Read the model definition and answer for the solid it produces. Units are mm, in the model's axes. A direction names the side the tool comes from. Give positions to 0.01 mm unless a question says otherwise; leave off trailing zeros. Loops run counter-clockwise (first coordinate to the right, second up) from the corner with the lowest first, then second, coordinate; pieces in that order, holes last.
(1) Find section C-C, the plane x = 1.5. Write down the section's boundary in (y, z), then the cut area to 3 significant figures.
(2) Find section A-A, the plane x = 6.75. Write down the section's boundary in (y, z), then the cut area to 3 significant figures.
(3) Straight lines are drawn through the part: probe 1 along Y at (x, z) = (15.95, 11.5); probe 2 along Z at (x, y) = (15.3, 10); probe 3 along X at (y, z) = (10, 4.2). For each, find the intervals that lie inside material, in ascending order.
(4) Each of these flat-tipped pins is pushed along its axis until it touches: P1, Ø6.5, axis at y = 11, z = 10, coming from the -X side; P2, Ø5.5, axis at y = 10, z = 11.5, coming from the -X side; P3, Ø4, axis at y = 6, z = 12.5, coming from the -X side. Where does it stop, or does it pass through?
(5) Find section B-B, the plane z = 4. Write down the section's boundary in (x, y).
(6) Determine the mould class of faces 1 (the face through (13.801, 0.285, 9.473)), 2 (the face through (13.5, 10, 15)), 3 (the face through (17, 12, 11)), 4 (the face through (17.21, 16.99, 18.65)) for opening direction Y: pulls with the +Y half, pulls with the -Y half, needs draft (parallel to the pull), parting line crosses it, or undercut.
(7) Which of the six approach directions +Z, -Z, +X, -X, +Y, -Y give full straight-line access (tool end or side, diameter ignored) to faces 5 (the face through (0.301, 9.874, 6.215)), 6 (the face through (5, 9, 3)), 7 (the face through (0.301, 19.715, 2.788)), 8 (the face through (6.67, 19.699, 6.215)), 9 (the face through (15.274, 9.875, 8.653))?
Autodesk Fusion 360 part; units mm, degrees
sketch "Sketch1" plane through (0, 0, 0) normal (0, 0, 1) x (1, 0, 0)
  line L0 (0, 0) -> (20, 0)
  line L1 (20, 0) -> (20, 20)
  line L2 (20, 20) -> (0, 20)
  line L3 (0, 20) -> (0, 0)
  dimension "d34" = 20
extrude "Extrude1" add sketch "Sketch1" along normal blind 6.5
sketch "Sketch2" plane through (0, 0, 6.5) normal (0, 0, 1) x (-1, 0, 0)
  line L0 (0, -20) -> (0, 0)
  line L1 (0, 0) -> (-20, 0)
  line L2 (-20, 0) -> (-20, -20)
  line L3 (-20, -20) -> (0, -20)
  line L4 (-20, -20) -> (-20, 0)
  line L5 (-13.5, 0) -> (-13.5, -20)
  line L6 (-13.5, -20) -> (0, 0) construction
  dimension "d33" = 6.5
extrude "Extrude2" add sketch "Sketch2" along normal blind 15 contours L1 L2 L3 L4 L5
sketch "Sketch5" plane through (20, 0, 0) normal (1, 0, 0) x (0, 1, 0)
  line L0 (0, 21.5) -> (0, 0)
  line L1 (0, 0) -> (20, 0)
  line L2 (20, 0) -> (20, 21.5)
  line L3 (20, 21.5) -> (0, 21.5)
  line L4 (0, 21.5) -> (20, 1.5) construction
  line L5 (0, 21.5) -> (20, 21.5) construction
  line L6 (20, 21.5) -> (10, 11.5) construction
  dimension "d37" = 45
fillet "Fillet2" radius 10 2 edges at (16.75, 20, 21.5) (16.75, 0, 21.5)
hole "Hole3" at (13.5, 10, 11.5) direction (1, 0, 0) diameter 3.5 end through all counterbore diameter 5.7 counterbore depth 3.5
hole "Hole4" at (6.75, 10, 6.5) direction (0, 0, -1) diameter 3.5 end through all counterbore diameter 5.7 counterbore depth 3.5
fillet "Fillet1" radius 1 9 edges at (0, 20, 3.25) (0, 0, 3.25) (6.75, 0, 6.5) (6.75, 20, 6.5) (0, 10, 6.5) (13.5, 20, 9) (13.5, 10, 21.5) (13.5, 0, 9) (13.5, 10, 6.5)
Entries:
1. outline: (0, 0) - (20, 0) - (20, 5.5) arc R1 ccw to (19, 6.5) - (1, 6.5) arc R1 ccw to (0, 5.5) - close
1. area: 130 mm2
2. outline: (0, 0) - (8.25, 0) - (8.25, 3) - (7.15, 3) - (7.15, 6.5) - (1, 6.5) arc R1 ccw to (0, 5.5) - close; (11.75, 0) - (20, 0) - (20, 5.5) arc R1 ccw to (19, 6.5) - (12.85, 6.5) - (12.85, 3) - (11.75, 3) - close
2. area: 99.1 mm2
3. probe 1: y = 0 to 7.15, 12.85 to 20
3. probe 2: z = 0 to 8.65, 14.35 to 21.5
3. probe 3: x = 0 to 3.9, 9.6 to 20
4. P1: stops at x = 13.16
4. P2: stops at x = 17
4. P3: stops at x = 13.5
5. outline: (0, 1) arc R1 ccw to (1, 0) - (20, 0) - (20, 20) - (1, 20) arc R1 ccw to (0, 19) - close; hole circle Ø5.7 at (6.75, 10)
6. face 1: pulls with the -Y half
6. face 2: needs draft
6. face 3: undercut
6. face 4: pulls with the +Y half
7. face 5: +Z, -X, +Y, -Y
7. face 6: +Z
7. face 7: +Z, -Z, -X, +Y
7. face 8: +Z, -X, +Y
7. face 9: -X
